Geometry: final body of the model. Coordinates: model frame, mm. Face numbers are marked on the shaded views. Round coordinates to 2 decimals unless told otherwise and drop trailing zeros. Order: outer loops, then holes, each group sorted by start corner. A loop starts at its lowest first (then second) coordinate and runs counter-clockwise, first axis right, second up. Notation, with made-up numbers: (-17, 79) -> (-1, 79) arc R19 ccw to (-1, 95) -> close; hole circle Ø2 at (-1.5, 6). An arc over 180 degrees is marked (long way). Put each result on its own line as item: value.
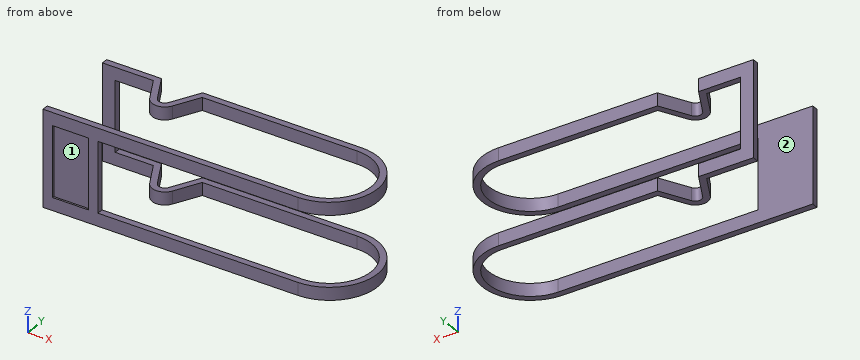
```python
from build123d import *

# Parameters (mm, degrees)
F1_DEPTH = 15
F2_W     = 7.4999995679
F2_H     = 11
F2_W_2   = 24.9287047806
F2_W_3   = 6.4644805853
F3_DEPTH = 25
F4_W     = 6.6068146341
F4_H     = 11
F5_DEPTH = 3
F6_W     = 5.6068146341
F6_H     = 11
F7_DEPTH = 0.3


with BuildPart() as f1:
    # F0 (on Top) → F1 (new body)
    with BuildSketch(Plane.XY):
        with BuildLine():
            Line((0, 0.9999995679), (0, 0))
            Line((0, 0), (40, 0))
            ThreePointArc((40, 0), (47.4999995679, 7.4999995679), (40, 14.9999991357))
            Line((40, 14.9999991357), (15.0712952194, 14.9999991357))
            Line((15.0712952194, 14.9999991357), (12.7260657599, 10.4948552605))
            ThreePointArc((12.7260657599, 10.4948552605), (11.8390549267, 9.9566038737), (10.9520440936, 10.4948552605))
            Line((10.9520440936, 10.4948552605), (8.6068146341, 14.9999991357))
            Line((8.6068146341, 14.9999991357), (0, 14.9999991357))
            Line((0, 14.9999991357), (0, 13.9999995679))
            Line((0, 13.9999995679), (8, 13.9999995679))
            Line((8, 13.9999995679), (10.0650336437, 10.0331068468))
            ThreePointArc((10.0650336437, 10.0331068468), (11.8390549267, 8.9566043058), (13.6130762098, 10.0331068468))
            Line((13.6130762098, 10.0331068468), (15.6781098535, 13.9999995679))
            Line((15.6781098535, 13.9999995679), (40, 13.9999995679))
            ThreePointArc((40, 13.9999995679), (46.5, 7.4999995679), (40, 0.9999995679))
            Line((40, 0.9999995679), (0, 0.9999995679))
        make_face()
    extrude(amount=F1_DEPTH)

    # F2 (on face) → F3 (cut)
    with BuildSketch(Plane(origin=(0, 14.9999991357, 0), x_dir=(-1, 0, 0), z_dir=(0, 1, 0))):
        with Locations((-43.7499997839, 7.5)):
            Rectangle(F2_W, F2_H)
        with Locations((-27.5356476097, 7.5)):
            Rectangle(F2_W_2, F2_H)
        with Locations((-11.8390549267, 7.5)):
            Rectangle(F2_W_3, F2_H)
    extrude(amount=-F3_DEPTH, mode=Mode.SUBTRACT)

    # F4 (on face) → F5 (cut)
    with BuildSketch(Plane(origin=(0, 14.9999991357, 0), x_dir=(-1, 0, 0), z_dir=(0, 1, 0))):
        with Locations((-5.303407317, 7.5)):
            Rectangle(F4_W, F4_H)
    extrude(amount=-F5_DEPTH, mode=Mode.SUBTRACT)

    # F6 (on face) → F7 (cut)
    with BuildSketch(Plane.XZ):
        with Locations((4.303407317, 7.5)):
            Rectangle(F6_W, F6_H)
    extrude(amount=-F7_DEPTH, mode=Mode.SUBTRACT)


solid = f1.part
```
1. Contact query for flat-ended pins moving along their axis: P1, Ø0.8, axis at y = 0.5, z = 7, coming from the +X side; P2, Ø1.7, axis at x = 4.5, z = 5.5, coming from the -Y side; P3, Ø6, axis at x = 29, y = 10.5, coming from the +Z side; P4, Ø1.1, axis at y = 14.5, z = 9, coming from the +X side. Output: stop coordinate, or through.
Ans:
P1: x = 8.61
P2: y = 0.3
P3: through
P4: x = 2
2. Draft query along Y for the marked faces 1 and 2. Return one class per face: +Y half, -Y half, draft (parallel to the pull), parting line (faces both ways), or undercut.
Ans:
face 1: -Y half
face 2: undercut
3. Cut plane B-B on x = 38. Return loops of the section in (y, z), and give its area (3 significant figures).
Ans:
outline: (0, 0) -> (1, 0) -> (1, 2) -> (0, 2) -> close; (0, 13) -> (1, 13) -> (1, 15) -> (0, 15) -> close; (14, 0) -> (15, 0) -> (15, 2) -> (14, 2) -> close; (14, 13) -> (15, 13) -> (15, 15) -> (14, 15) -> close
area: 8.00 mm²
4. Cut plane C-C on x = 5.5. Return loops of the section in (y, z), and give its area (3 significant figures).
Ans:
outline: (0, 0) -> (1, 0) -> (1, 15) -> (0, 15) -> (0, 13) -> (0.3, 13) -> (0.3, 2) -> (0, 2) -> close; (14, 0) -> (15, 0) -> (15, 2) -> (14, 2) -> close; (14, 13) -> (15, 13) -> (15, 15) -> (14, 15) -> close
area: 15.7 mm²
5. Material intervals for probe 1 along Y at (x, z) = (19, 13.5); probe 2 along X at (y, z) = (14.75, 5.5); probe 3 along X at (y, z) = (10.5, 14), sorted ascending.
Ans:
probe 1: 0 to 1, 14 to 15
probe 2: 0 to 2
probe 3: 9.82 to 10.95, 12.73 to 13.86, 45.77 to 46.87
6. Cut plane A-A on z = 8. Return loops of the section in (x, y), and give its area (3 significant figures).
Ans:
outline: (0, 0) -> (1.5, 0) -> (1.5, 0.3) -> (7.11, 0.3) -> (7.11, 0) -> (8.61, 0) -> (8.61, 1) -> (0, 1) -> close; (0, 14) -> (2, 14) -> (2, 15) -> (0, 15) -> close
area: 8.92 mm²
7. Cut plane D-D on y = 5.75. Return loops of the section in (x, z), and give its area (3 significant figures).
Ans:
outline: (46.26, 0) -> (47.29, 0) -> (47.29, 2) -> (46.26, 2) -> close; (46.26, 13) -> (47.29, 13) -> (47.29, 15) -> (46.26, 15) -> close
area: 4.13 mm²
